```python
from build123d import *

# Parameters (mm, degrees)
F1_DEPTH = 25
F2_R     = 17
F3_DEPTH = 10


with BuildPart() as f1:
    # F0 (on Front) → F1 (new body, symmetric)
    with BuildSketch(Plane.XZ):
        Polygon((-10, 0), (0, 0), (0, 53), (0, 66), (-10, 66), align=None)
        with BuildLine():
            Line((0, 66), (0, 53))
            ThreePointArc((0, 53), (3, 56), (6, 53))
            Line((6, 53), (6, 66))
            Line((6, 66), (0, 66))
        make_face()
        Polygon((6, 66), (6, 53), (6, 48), (11, 48), (11, 66), align=None)
    extrude(amount=F1_DEPTH, both=True)

    # F2 (on face) → F3 (cut, through all)
    with BuildSketch(Plane(origin=(-10, 0, 0), x_dir=(0, -1, 0), z_dir=(-1, 0, 0))):
        with Locations((0, 27)):
            Circle(F2_R)
    extrude(amount=-F3_DEPTH, mode=Mode.SUBTRACT)


solid = f1.part
```
Read the model definition and answer for the solid it produces. Units are mm, in the model's axes. A direction names the side the tool comes from. Give positions to 0.01 mm unless a question says otherwise; leave off trailing zeros. Order: outer loops, then holes, each group sorted by start corner. A loop starts at its lowest first (then second) coordinate and runs counter-clockwise, first axis right, second up. Notation, with made-up numbers: (48.25, 16.5) -> (81.25, 16.5) arc R10 ccw to (81.25, 34.5) -> close; hole circle Ø3 at (42, 80.5). An arc over 180 degrees is marked (long way). Write item = value, one per line.
1. Given pin 1 (1.5 mm diameter, centred on x = 9, y = -7, fed in from -Z); pin 2 (25 mm diameter, centred on y = 11.5, z = 21.5, fed in from +X), each flat-ended and moving along its own axis, determine where each tip first touches the part or whether it passes through.
Numbers:
pin_1 = 48
pin_2 = 0
2. A cutting plane is placed at D-D, the plane y = -20. Write down the section's boundary in (x, z), and give its area (3 significant figures).
Numbers:
outline = (-10, 0) -> (0, 0) -> (0, 53) arc R3 cw to (6, 53) -> (6, 48) -> (11, 48) -> (11, 66) -> (-10, 66) -> close
area = 814 mm²
3. A cutting plane is placed at A-A, the plane y = 8. Write down the section's boundary in (x, z), and give its area (3 significant figures).
Numbers:
outline = (-10, 0) -> (0, 0) -> (0, 12) -> (-10, 12) -> close; (-10, 42) -> (0, 42) -> (0, 53) arc R3 cw to (6, 53) -> (6, 48) -> (11, 48) -> (11, 66) -> (-10, 66) -> close
area = 514 mm²
4. A cutting plane is placed at C-C, the plane x = -3.25. Write down the section's boundary in (y, z), and give its area (3 significant figures).
Numbers:
outline = (-25, 0) -> (25, 0) -> (25, 66) -> (-25, 66) -> close; hole circle Ø34 at (0, 27)
area = 2,390 mm²
5. For faces 1 (the face through (-10, -11, 41)), 2 (the face through (0, -17, 20)), 3 (the face through (8, 0, 48)), determine the directions among +Z, -Z, +X, -X, +Y, -Y from which every point of the face is accessible in a straight line to the end or side of a thin tool.
Numbers:
face_1 = +Z, -Z, -X, +Y, -Y
face_2 = -Z, +Y, -Y
face_3 = -Z, +X, +Y, -Y
6. A cutting plane is placed at B-B, the plane z = 27. Write down the section's boundary in (x, y), and give its area (3 significant figures).
Numbers:
outline = (-10, -25) -> (0, -25) -> (0, -17) -> (-10, -17) -> close; (-10, 17) -> (0, 17) -> (0, 25) -> (-10, 25) -> close
area = 160 mm²
7. Straight lines are drawn through the part: line 1 along Z through (x, y) = (-2.5, 0); line 2 along X through (y, z) = (-9.5, 50.5); line 3 along Z through (x, y) = (9.5, 1.5). For each, find the intervals that lie inside material, in ascending order.
Numbers:
line_1 = 0 to 10, 44 to 66
line_2 = -10 to 0, 6 to 11
line_3 = 48 to 66
8. The mould has two halves that part along X. Classify faces 4 (the face through (3, 0, 56)), 5 (the face through (-2, 25, 41)), 6 (the face through (11, 0, 57)): +X half, -X half, draft (parallel to the pull), parting line (faces both ways), or undercut.
Numbers:
face_4 = undercut
face_5 = draft
face_6 = +X half
